Design review of the part built by this model. Coordinates are the model's own, in mm. Face numbers are marked on the shaded views. Round coordinates to 2 decimals unless told otherwise and drop trailing zeros. Order: outer loops, then holes, each group sorted by start corner. A loop starts at its lowest first (then second) coordinate and runs counter-clockwise, first axis right, second up. Notation, with made-up numbers: M -5,35 L 27,35 A15 cw 27,49 Z; hole C -27,29 d6. An arc over 180 degrees is marked long. Use a Markdown table: item, result. Add a question column.
(1) Take a section at B-B (y = 113.5). Write out the cut boundary in (x, z), then the cut area to 3 significant figures.
(2) To check wall thickness, follow probe 1 along Z at (x, y) = (-15.52, 8.75); probe 2 along Z at (x, y) = (12.75, 210); probe 3 along Z at (x, y) = (15, 5). State the ranges of each line that lie inside material, in increasing order. Write a range as from..to.
(3) For pin 1 (1.5 mm diameter, centred on x = -30, z = -10, fed in from +Y); pin 2 (3 mm diameter, centred on y = 40.5, z = 52.5, fed in from -X); pin 3 (4.5 mm diameter, centred on x = -58, z = 5.5, fed in from +Y); pin 4 (3 mm diameter, centred on x = -30, z = 0, fed in from -Y), all flat-tipped, find the tip position at first contact; note any pin that passes through.
(4) Take a section at A-A (y = 194). Write out the cut boundary in (x, z).
(5) The part is to be moulded in two halves that separate along Z. For the marked faces 1, 2 and 3, say which applies: released by +Z, released by -Z, zero draft, split by the parting line, or undercut.
(6) Take a section at C-C (y = 21.5). Write out the cut boundary in (x, z), then the cut area to 3 significant figures.
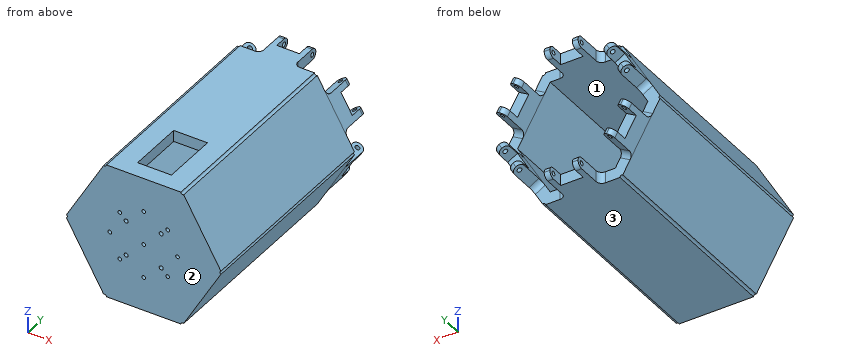
```python
from build123d import *

# Parameters (mm, degrees)
BOSS_EXTRUDE1_DEPTH                 = 15
BOSS_EXTRUDE3_DEPTH                 = 170
SKETCH5_W                           = 30
SKETCH5_H                           = 10
BOSS_EXTRUDE4_DEPTH                 = 30
CIRPATTERN2_COUNT                   = 6
CUT_EXTRUDE1_REACH                  = 264.726
SKETCH7_W                           = 20
SKETCH7_H                           = 15
CIRPATTERN4_COUNT                   = 6
FILLET1_R                           = 5
F_4_0_MM_DOWEL_HOLES1_D             = 4
CIRPATTERN8_COUNT                   = 6
CUT_EXTRUDE2_REACH                  = 257.783
SKETCH11_W                          = 30
SKETCH11_H                          = 50
M3_CLEARANCE_HOLE1_D                = 3.6
LPATTERN1_COUNT                     = 2
LPATTERN1_PITCH                     = 31.04
LPATTERN1_COUNT_DIR2                = 2
LPATTERN1_PITCH_DIR2                = 31.04
TAP_DRILL_FOR_M4X0_7_TAP2_OUTLINE_R = 1.65
TAP_DRILL_FOR_M4X0_7_TAP2_DEPTH     = 185


# Read off the part's stored shape, not the designer's step: Tap Drill for M4x0.7 Tap2
with BuildPart() as part:
    # Sketch1 → Boss-Extrude1 (new body)
    with BuildSketch(Plane(origin=(0, 0, 0), x_dir=(1, 0, 0), z_dir=(0, 1, 0))):
        Polygon((-69.282032303, 0), (-34.641016151, 60), (34.641016151, 60), (69.282032303, 0), (34.641016151, -60), (-34.641016151, -60), align=None)
    extrude(amount=BOSS_EXTRUDE1_DEPTH)

    # Sketch4 → Boss-Extrude3 (add)
    with BuildSketch(Plane(origin=(0, 15, 0), x_dir=(1, 0, 0), z_dir=(0, 1, 0))):
        Polygon((-34.641016151, -60), (34.641016151, -60), (69.282032303, 0), (57.735026919, 0), (28.867513459, -50), (-28.867513459, -50), (-57.735026919, 0), (-69.282032303, 0), align=None)
    boss_extrude3 = extrude(amount=BOSS_EXTRUDE3_DEPTH)

    # Mirror1: Boss-Extrude3 across plane
    add(boss_extrude3.mirror(Plane(origin=(57.735026919, 185, 0), x_dir=(1, 0, 0), z_dir=(0, 0, 1))))

    # Sketch5 → Boss-Extrude4 (add)
    with BuildSketch(Plane(origin=(0, 185, 0), x_dir=(1, 0, 0), z_dir=(0, 1, 0))):
        with Locations((0, -55)):
            Rectangle(SKETCH5_W, SKETCH5_H)
    boss_extrude4 = extrude(amount=BOSS_EXTRUDE4_DEPTH)

    # CirPattern2: Boss-Extrude4 ×6 about axis
    cirpattern2_axis = Axis((0, 0, 0), (0, 1, 0))
    for i in range(1, CIRPATTERN2_COUNT):
        add(boss_extrude4.rotate(cirpattern2_axis, i * 360 / CIRPATTERN2_COUNT))

    # Sketch7 → Cut-Extrude1 (cut, up to next)
    with BuildSketch(Plane(origin=(-51.961524227, 0, 30), x_dir=(0.49999999999999695, 0, 0.8660254037844404), z_dir=(-0.8660254037844404, 0, 0.49999999999999695)), mode=Mode.PRIVATE) as cut_extrude1_sk1:
        with Locations((0, 207.5)):
            Rectangle(SKETCH7_W, SKETCH7_H)
    cut_extrude1_tool1 = extrude(cut_extrude1_sk1.sketch, amount=-CUT_EXTRUDE1_REACH, mode=Mode.PRIVATE) & part.part
    cut_extrude1 = cut_extrude1_tool1.solids().sort_by_distance((-51.961524, 207.5, 30))[0]
    add(cut_extrude1, mode=Mode.SUBTRACT)

    # CirPattern4: Cut-Extrude1 ×6 about axis
    cirpattern4_axis = Axis((0, 0, 0), (0, 1, 0))
    for i in range(1, CIRPATTERN4_COUNT):
        add(cut_extrude1.rotate(cirpattern4_axis, i * 360 / CIRPATTERN4_COUNT), mode=Mode.SUBTRACT)

    # Fillet1
    fillet1_edges = [part.edges().sort_by_distance(p)[0] for p in [
        (-55.131397208, 185, 14.509618943),
        (-40.131397208, 185, 40.490381057),
        (-40.131397208, 185, -40.490381057),
        (-55.131397208, 185, -14.509618943),
        (15, 185, -55),
        (-15, 185, -55),
        (55.131397208, 185, -14.509618943),
        (40.131397208, 185, -40.490381057),
        (40.131397208, 185, 40.490381057),
        (55.131397208, 185, 14.509618943),
        (-15, 185, 55),
        (15, 185, 55),
    ]]
    fillet(fillet1_edges, radius=FILLET1_R)
    fillet1_2_edges = [part.edges().sort_by_distance(p)[0] for p in [
        (-49.551270189, 215, 14.174682453),
        (-58.211524227, 215, 19.174682453),
        (-37.051270189, 215, -35.825317547),
        (-45.711524227, 215, -40.825317547),
        (12.5, 215, -50),
        (12.5, 215, -60),
        (49.551270189, 215, -14.174682453),
        (58.211524227, 215, -19.174682453),
        (37.051270189, 215, 35.825317547),
        (45.711524227, 215, 40.825317547),
        (-37.051270189, 215, 35.825317547),
        (-45.711524227, 215, 40.825317547),
        (49.551270189, 215, 14.174682453),
        (58.211524227, 215, 19.174682453),
        (-49.551270189, 215, -14.174682453),
        (-58.211524227, 215, -19.174682453),
        (-12.5, 215, -50),
        (-12.5, 215, -60),
        (37.051270189, 215, -35.825317547),
        (45.711524227, 215, -40.825317547),
        (12.5, 215, 50),
        (12.5, 215, 60),
        (-12.5, 215, 50),
        (-12.5, 215, 60),
    ]]
    fillet(fillet1_2_edges, radius=FILLET1_R - 0.0001)  # a hair under: the kernel refuses the full size

    # Ø4.0 mm Dowel Holes1 (through all)
    with Locations(Plane(origin=(15, 0, 0), x_dir=(0, 0, -1), z_dir=(1, 0, 0))):
        with Locations((-55, 210)):
            f_4_0_mm_dowel_holes1 = Hole(F_4_0_MM_DOWEL_HOLES1_D / 2)

    # CirPattern8: Ø4.0 mm Dowel Holes1 ×6 about axis
    cirpattern8_axis = Axis((0, 15, 0), (0, -1, 0))
    for i in range(1, CIRPATTERN8_COUNT):
        add(f_4_0_mm_dowel_holes1.rotate(cirpattern8_axis, i * 360 / CIRPATTERN8_COUNT), mode=Mode.SUBTRACT)

    # Sketch11 → Cut-Extrude2 (cut, up to next)
    with BuildSketch(Plane.XY.offset(60), mode=Mode.PRIVATE) as cut_extrude2_sk1:
        with Locations((0, 40)):
            Rectangle(SKETCH11_W, SKETCH11_H)
    cut_extrude2_tool1 = extrude(cut_extrude2_sk1.sketch, amount=-CUT_EXTRUDE2_REACH, mode=Mode.PRIVATE) & part.part
    add(cut_extrude2_tool1.solids().sort_by_distance((0, 40, 60))[0], mode=Mode.SUBTRACT)

    # M3 Clearance Hole1 (through all)
    with Locations(Plane(origin=(0, 0, 0), x_dir=(-1, 0, 0), z_dir=(0, -1, 0))):
        with Locations((-15.52, 15.52)):
            m3_clearance_hole1 = Hole(M3_CLEARANCE_HOLE1_D / 2)

    # LPattern1: M3 Clearance Hole1 2 × 2
    with Locations(*[(-i * LPATTERN1_PITCH, 0, j * LPATTERN1_PITCH_DIR2) for i in range(LPATTERN1_COUNT) for j in range(LPATTERN1_COUNT_DIR2) if (i, j) != (0, 0)]):
        add(m3_clearance_hole1, mode=Mode.SUBTRACT)

    # Tap Drill for M4x0.7 Tap2 outline → Tap Drill for M4x0.7 Tap2 (cut)
    with BuildSketch(Plane(origin=(0, 0, 0), x_dir=(1, 0, 0), z_dir=(0, 1, 0))):
        Circle(TAP_DRILL_FOR_M4X0_7_TAP2_OUTLINE_R)
        with Locations((-21.213203436, -21.213203436)):
            Circle(TAP_DRILL_FOR_M4X0_7_TAP2_OUTLINE_R)
        with Locations((-30, 0)):
            Circle(TAP_DRILL_FOR_M4X0_7_TAP2_OUTLINE_R)
        with Locations((-21.213203436, 21.213203436)):
            Circle(TAP_DRILL_FOR_M4X0_7_TAP2_OUTLINE_R)
        with Locations((0, 30)):
            Circle(TAP_DRILL_FOR_M4X0_7_TAP2_OUTLINE_R)
        with Locations((21.213203436, 21.213203436)):
            Circle(TAP_DRILL_FOR_M4X0_7_TAP2_OUTLINE_R)
        with Locations((30, 0)):
            Circle(TAP_DRILL_FOR_M4X0_7_TAP2_OUTLINE_R)
        with Locations((21.213203436, -21.213203436)):
            Circle(TAP_DRILL_FOR_M4X0_7_TAP2_OUTLINE_R)
        with Locations((0, -30)):
            Circle(TAP_DRILL_FOR_M4X0_7_TAP2_OUTLINE_R)
        with BuildLine():
            ThreePointArc((-32.991016151, -60), (-33.816016151, -58.571058084), (-35.466016151, -58.571058084))
            Line((-35.466016151, -58.571058084), (-34.641016151, -60))
            Line((-34.641016151, -60), (-32.991016151, -60))
        make_face()
        with BuildLine():
            Line((-69.282032303, 0), (-68.457032303, -1.428941916))
            ThreePointArc((-68.457032303, -1.428941916), (-67.632032303, 0), (-68.457032303, 1.428941916))
            Line((-68.457032303, 1.428941916), (-69.282032303, 0))
        make_face()
        with BuildLine():
            ThreePointArc((35.466016151, -58.571058084), (33.816016151, -58.571058084), (32.991016151, -60))
            Line((32.991016151, -60), (34.641016151, -60))
            Line((34.641016151, -60), (35.466016151, -58.571058084))
        make_face()
        with BuildLine():
            Line((-34.641016151, 60), (-35.466016151, 58.571058084))
            ThreePointArc((-35.466016151, 58.571058084), (-33.816016151, 58.571058084), (-32.991016151, 60))
            Line((-32.991016151, 60), (-34.641016151, 60))
        make_face()
        with BuildLine():
            ThreePointArc((68.457032303, 1.428941916), (67.632032303, 0), (68.457032303, -1.428941916))
            Line((68.457032303, -1.428941916), (69.282032303, 0))
            Line((69.282032303, 0), (68.457032303, 1.428941916))
        make_face()
        with BuildLine():
            Line((34.641016151, 60), (32.991016151, 60))
            ThreePointArc((32.991016151, 60), (33.816016151, 58.571058084), (35.466016151, 58.571058084))
            Line((35.466016151, 58.571058084), (34.641016151, 60))
        make_face()
    extrude(amount=TAP_DRILL_FOR_M4X0_7_TAP2_DEPTH, mode=Mode.SUBTRACT)


solid = part.part
```
Verdict:
| question | item | result |
|---|---|---|
| 1 | outline | M -68.46,-1.43 L -35.47,-58.57 A1.65 cw -32.99,-60 L 32.99,-60 A1.65 cw 35.47,-58.57 L 68.46,-1.43 A1.65 cw 68.46,1.43 L 35.47,58.57 A1.65 cw 32.99,60 L -32.99,60 A1.65 cw -35.47,58.57 L -68.46,1.43 A1.65 cw Z; hole M -57.74,0 L -28.87,-50 L 28.87,-50 L 57.74,0 L 28.87,50 L -28.87,50 Z |
| 1 | area | 3,790 mm^2 |
| 2 | probe 1 | z = -60..-17.32, -13.72..13.72, 17.32..60 |
| 2 | probe 2 | z = -60..-57, -53..-50, 50..53, 57..60 |
| 2 | probe 3 | z = -60..-17.24, -13.8..13.8, 17.24..60 |
| 3 | pin 1 | stops at y = 15 |
| 3 | pin 2 | stops at x = -39.84 |
| 3 | pin 3 | stops at y = 185 |
| 3 | pin 4 | passes through |
| 4 | outline | M -59.46,-17.01 L -44.46,-42.99 L -35.8,-37.99 L -50.8,-12.01 Z; M -59.46,17.01 L -50.8,12.01 L -35.8,37.99 L -44.46,42.99 Z; M -15,-60 L 15,-60 L 15,-50 L -15,-50 Z; M -15,50 L 15,50 L 15,60 L -15,60 Z; M 35.8,-37.99 L 44.46,-42.99 L 59.46,-17.01 L 50.8,-12.01 Z; M 35.8,37.99 L 50.8,12.01 L 59.46,17.01 L 44.46,42.99 Z |
| 5 | face 1 | undercut |
| 5 | face 2 | zero draft |
| 5 | face 3 | released by -Z |
| 6 | outline | M -68.46,-1.43 L -35.47,-58.57 A1.65 cw -32.99,-60 L 32.99,-60 A1.65 cw 35.47,-58.57 L 68.46,-1.43 A1.65 cw 68.46,1.43 L 35.47,58.57 A1.65 cw 32.99,60 L 15,60 L 15,50 L 28.87,50 L 57.74,0 L 28.87,-50 L -28.87,-50 L -57.74,0 L -28.87,50 L -15,50 L -15,60 L -32.99,60 A1.65 cw -35.47,58.57 L -68.46,1.43 A1.65 cw Z |
| 6 | area | 3,490 mm^2 |
